from build123d import *

# Parameters (mm, degrees)
SKETCH1_W           = 88.9
SKETCH1_H           = 127
BOSS_EXTRUDE1_DEPTH = 355.6
FILLET1_R           = 31.75
SKETCH3_W           = 88.9
SKETCH3_H           = 127
BOSS_EXTRUDE2_DEPTH = 495.3
FILLET2_R           = 31.75


# Read off the part's stored shape, not the designer's step: Mirror1
with BuildPart() as part:
    # Sketch1 → Boss-Extrude1 (new, symmetric)
    with BuildSketch(Plane(origin=(0, 0, 0), x_dir=(0, 0, -1), z_dir=(1, 0, 0))):
        Rectangle(SKETCH1_W, SKETCH1_H)
    extrude(amount=BOSS_EXTRUDE1_DEPTH, both=True)

    # Fillet1
    fillet1_edges = [part.edges().sort_by_distance(p)[0] for p in [
        (0, -63.5, -44.45),
        (0, 63.5, -44.45),
    ]]
    fillet(fillet1_edges, radius=FILLET1_R)

    # Sketch3 → Boss-Extrude2 (add)
    with BuildSketch(Plane(origin=(0, 0, -44.45), x_dir=(-1, 0, 0), z_dir=(0, 0, -1))):
        with Locations((400.05, 0)):
            Rectangle(SKETCH3_W, SKETCH3_H)
    extrude(amount=-BOSS_EXTRUDE2_DEPTH)

    # Fillet2
    fillet2_edges = [part.edges().sort_by_distance(p)[0] for p in [
        (-400.05, -63.5, -44.45),
        (-400.05, 63.5, -44.45),
        (-444.5, 0, -44.45),
        (-444.5, -63.5, 203.2),
        (-444.5, 63.5, 203.2),
    ]]
    fillet(fillet2_edges, radius=FILLET2_R)

    # Mirror1: part across plane


with BuildPart() as part_1:
    add(part.part)
    add(part.part.mirror(Plane(origin=(0, 0, 0), x_dir=(0, 0, 1), z_dir=(1, 0, 0))))


solid = part_1.part
Could you check a few things on this model? Use its own coordinates, in mm. A direction names the side the tool comes from. Coordinates: 2 decimals unless noted, no trailing zeros. Write each loop counter-clockwise with the first axis right and the second up, starting at its lowest first coordinate (ties: lowest second). Pieces come first, ordered by that corner, then holes. Notation, with made-up numbers: (21, -23) - (73, -23) arc R20 cw to (73, -12) - close; hole circle Ø2 at (-32, 67.25). An arc over 180 degrees is marked (long way). Put each result on its own line as item: value. Start each with the question number.
Q1. I'm going to push a flat-ended pin straight in: P1, Ø1, axis at x = 144, y = -9.5, coming from the +Z side. Where does the tip first touch, or does it pass through?
Q2. I want a section at C-C on x = -329.5. Write out the boundary of the cut face in (y, z).
Q3. Please list where these lines run through material, in increasing order: L1, parallel to X at y = -22.5, z = 240; L2, parallel to Z at x = -54.5, y = 32; L3, parallel to Z at x = -40, y = -35.
Q4. I want a section at D-D on y = -53. Write out the boundary of the cut face in (x, z).
Q5. Thinking about a two-plate mould opening in X: for faces 1 (the cylindrical face through (-435.4, 54, 222.3)), 2 (the cylindrical face through (434.95, 0.44, -35.4)), 3 (the flat face through (-355.6, -1, 245)), 4 (the flat face through (355.6, -1, 245)), which applies, pulls with the +X half, pulls with the -X half, needs draft (parallel to the pull), parting line crosses it, or undercut?
Q6. I want a section at A-A on z = 260.5. Write out the boundary of the cut face in (x, y).
Q7. I want a section at B-B on y = 22.5. Write out the boundary of the cut face in (x, z), plus the area to 3 significant figures.
Q8. Which directions (+Z, -Z, +X, -X, +Y, -Y) give clear straight access to the entire face, cutting with the end or side of a thin tool? Please do faces 5 (the flat face through (-2, -63.5, 29)), 6 (the flat face through (5, -1, 44.45)).
Checks:
1. P1: z = 44.45
2. outline: (-63.5, -12.7) arc R31.75 ccw to (-31.75, -44.45) - (31.75, -44.45) arc R31.75 ccw to (63.5, -12.7) - (63.5, 44.45) - (-63.5, 44.45) - close
3. L1: -444.5 to -355.6, 355.6 to 444.5
3. L2: -44.45 to 44.45
3. L3: -44.28 to 44.45
4. outline: (-436.34, -12.7) arc R23.59 ccw to (-412.75, -36.29) - (412.75, -36.29) arc R23.59 ccw to (436.34, -12.7) - (436.34, 450.85) - (355.6, 450.85) - (355.6, 44.45) - (-355.6, 44.45) - (-355.6, 450.85) - (-436.34, 450.85) - close
5. face 1: pulls with the -X half
5. face 2: pulls with the +X half
5. face 3: undercut
5. face 4: undercut
6. outline: (-444.5, -31.75) arc R31.75 ccw to (-412.75, -63.5) - (-355.6, -63.5) - (-355.6, 63.5) - (-412.75, 63.5) arc R31.75 ccw to (-444.5, 31.75) - close; (355.6, -63.5) - (412.75, -63.5) arc R31.75 ccw to (444.5, -31.75) - (444.5, 31.75) arc R31.75 ccw to (412.75, 63.5) - (355.6, 63.5) - close
7. outline: (-444.5, -12.7) arc R31.75 ccw to (-412.75, -44.45) - (412.75, -44.45) arc R31.75 ccw to (444.5, -12.7) - (444.5, 450.85) - (355.6, 450.85) - (355.6, 44.45) - (-355.6, 44.45) - (-355.6, 450.85) - (-444.5, 450.85) - close
7. area: 151,000 mm²
8. face 5: +Z, -Z, +X, -X, -Y
8. face 6: +Z, +Y, -Y
